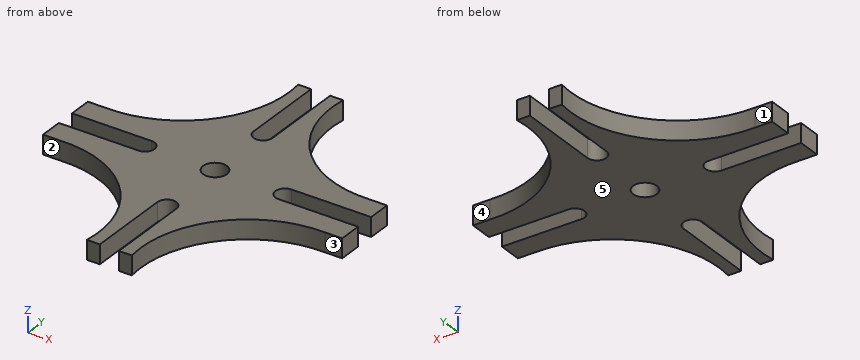
```python
from build123d import *

# Parameters (mm, degrees)
F1_DEPTH = 6.35
F2_R     = 3.96875
F3_DEPTH = 45.73795


with BuildPart() as f1:
    # F0 (on Top) → F1 (new body)
    with BuildSketch(Plane.XY):
        with BuildLine():
            ThreePointArc((-7.484571, 51.258114), (-16.386664, 22.501379), (-44.15456, 10.876361))
            Line((-44.15456, 10.876361), (-49.865723, 10.876361))
            Line((-49.865723, 10.876361), (-49.865723, 3.175))
            Line((-49.865723, 3.175), (-23.336682, 3.175))
            ThreePointArc((-23.336682, 3.175), (-20.161682, 0), (-23.336682, -3.175))
            Line((-23.336682, -3.175), (-49.865723, -3.175))
            Line((-49.865723, -3.175), (-49.865723, -10.876361))
            Line((-49.865723, -10.876361), (-44.15456, -10.876361))
            ThreePointArc((-44.15456, -10.876361), (-16.386664, -22.501379), (-7.484571, -51.258114))
            Line((-7.484571, -51.258114), (-3.175, -51.258114))
            Line((-3.175, -51.258114), (-3.175, -23.3426))
            ThreePointArc((-3.175, -23.3426), (0, -20.1676), (3.175, -23.3426))
            Line((3.175, -23.3426), (3.175, -51.258114))
            Line((3.175, -51.258114), (7.484571, -51.258114))
            ThreePointArc((7.484571, -51.258114), (16.386664, -22.501379), (44.15456, -10.876361))
            Line((44.15456, -10.876361), (49.865723, -10.876361))
            Line((49.865723, -10.876361), (49.865723, -3.175))
            Line((49.865723, -3.175), (23.336682, -3.175))
            ThreePointArc((23.336682, -3.175), (20.161682, 0), (23.336682, 3.175))
            Line((23.336682, 3.175), (49.865723, 3.175))
            Line((49.865723, 3.175), (49.865723, 10.876361))
            Line((49.865723, 10.876361), (44.15456, 10.876361))
            ThreePointArc((44.15456, 10.876361), (16.386664, 22.501379), (7.484571, 51.258114))
            Line((7.484571, 51.258114), (3.175, 51.258114))
            Line((3.175, 51.258114), (3.175, 23.3426))
            ThreePointArc((3.175, 23.3426), (0, 20.1676), (-3.175, 23.3426))
            Line((-3.175, 23.3426), (-3.175, 51.258114))
            Line((-3.175, 51.258114), (-7.484571, 51.258114))
        make_face()
    extrude(amount=F1_DEPTH)

    # F2 (on face) → F3 (cut)
    with BuildSketch(Plane(origin=(0, 0, 0), x_dir=(1, 0, 0), z_dir=(0, 0, -1))):
        Circle(F2_R)
    extrude(amount=-F3_DEPTH, mode=Mode.SUBTRACT)


solid = f1.part
```
Input: part model. Units: mm. Frame: model coordinates. Face numbers are marked on the shaded views. A direction names the side the tool comes from. Coordinates: 2 decimals unless noted, no trailing zeros. Loops run counter-clockwise (first coordinate to the right, second up) from the corner with the lowest first, then second, coordinate; pieces in that order, holes last. Notation, with made-up numbers: (-33, 54.5) - (13, 54.5) arc R28 ccw to (13, 73.5) - close; hole circle Ø11 at (-39.5, -24). An arc over 180 degrees is marked (long way). Answer in a Markdown table with one row per item.
(1) Set-up query: the marked faces 1, 2, 3, 4 and 5. Return all of +Z, -Z, +X, -X, +Y, -Y with unobstructed straight access to the full face (end or side cutting, diameter ignored); none if empty.
Model answer:
| item | result |
|---|---|
| face 1 | +Z, -Z, -X, +Y |
| face 2 | +Z, -Z, -X, -Y |
| face 3 | +Z, -Z, +X, -Y |
| face 4 | +Z, -Z, +X, +Y |
| face 5 | -Z, +X, -X, +Y, -Y |
(2) Cut plane D-D on x = -18.5. Output: boundary loops of the cut face in (y, z), plus the area to 3 significant figures.
Model answer:
| item | result |
|---|---|
| outline | (-20.36, 0) - (20.36, 0) - (20.36, 6.35) - (-20.36, 6.35) - close |
| area | 259 mm² |
(3) Cut plane C-C on y = 0. Output: boundary loops of the cut face in (x, z), plus the area to 3 significant figures.
Model answer:
| item | result |
|---|---|
| outline | (-20.16, 0) - (-3.97, 0) - (-3.97, 6.35) - (-20.16, 6.35) - close; (3.97, 0) - (20.16, 0) - (20.16, 6.35) - (3.97, 6.35) - close |
| area | 206 mm² |
(4) Cut plane A-A on x = 0. Output: boundary loops of the cut face in (y, z), plus the area to 3 significant figures.
Model answer:
| item | result |
|---|---|
| outline | (-20.17, 0) - (-3.97, 0) - (-3.97, 6.35) - (-20.17, 6.35) - close; (3.97, 0) - (20.17, 0) - (20.17, 6.35) - (3.97, 6.35) - close |
| area | 206 mm² |
(5) Pin query (flat end, axial travel): P1, Ø2, axis at x = -29, z = 5, coming from the +Y side; P2, Ø1.7, axis at x = 46, z = 3, coming from the -Y side; P3, Ø3, axis at x = -32, z = 2.5, coming from the +Y side. Return the tip coordinate at first contact, or that it passes through.
Model answer:
| item | result |
|---|---|
| P1 | stops at y = 14.03 |
| P2 | stops at y = -10.88 |
| P3 | stops at y = 13.01 |
(6) Material intervals for L1, parallel to Y at x = 0, z = 3.75; L2, parallel to X at y = 0, z = 5; L3, parallel to Y at x = -41, z = 4.5 (3 decimals), sorted ascending. Write a range as from..to.
Model answer:
| item | result |
|---|---|
| L1 | y = -20.17..-3.97, 3.97..20.17 |
| L2 | x = -20.16..-3.97, 3.97..20.16 |
| L3 | y = -10.888..-3.175, 3.175..10.888 |
